```python
from build123d import *

# Parameters (mm, degrees)
SALIENTE_EXTRUIR1_DEPTH = 10
REDONDEO1_R             = 10
REDONDEO2_R             = 10
CROQUIS2_R              = 2
CORTAR_EXTRUIR1_DEPTH   = 10


with BuildPart() as part:
    # Croquis1 → Saliente-Extruir1 (new body)
    with BuildSketch(Plane.XY):
        with BuildLine():
            Line((-15.183023411, 0), (15.183023411, 0))
            ThreePointArc((15.183023411, 0), (22.254091223, -2.928932188), (25.183023411, -10))
            Line((25.183023411, -10), (25.183023411, -16))
            ThreePointArc((25.183023411, -16), (22.254091223, -23.071067812), (15.183023411, -26))
            Line((15.183023411, -26), (12.183023411, -26))
            Line((12.183023411, -26), (12.183023411, -33))
            Line((12.183023411, -33), (25.183023411, -33))
            Line((25.183023411, -33), (32.183023411, -33))
            Line((32.183023411, -33), (32.183023411, 7))
            Line((32.183023411, 7), (32.183023411, 29.676278345))
            Line((32.183023411, 29.676278345), (19.078273373, 35.787123646))
            Line((19.078273373, 35.787123646), (16.119945541, 29.442969137))
            Line((16.119945541, 29.442969137), (25.183023411, 25.216786519))
            Line((25.183023411, 25.216786519), (23.183023411, 20.927772678))
            Line((23.183023411, 20.927772678), (25.183023411, 20.927772678))
            Line((25.183023411, 20.927772678), (25.183023411, 12))
            ThreePointArc((25.183023411, 12), (23.718557317, 8.464466094), (20.183023411, 7))
            Line((20.183023411, 7), (18.68839635, 7))
            Line((18.68839635, 7), (18.68839635, 11.289013841))
            Line((18.68839635, 11.289013841), (16.68839635, 7))
            Line((16.68839635, 7), (12.399382509, 9))
            Line((12.399382509, 9), (12.399382509, 7))
            Line((12.399382509, 7), (-15.183023411, 7))
            ThreePointArc((-15.183023411, 7), (-22.254091223, 9.928932188), (-25.183023411, 17))
            Line((-25.183023411, 17), (-25.183023411, 20.524963692))
            ThreePointArc((-25.183023411, 20.524963692), (-24.011450536, 23.353390817), (-21.183023411, 24.524963692))
            Line((-21.183023411, 24.524963692), (-20.89400957, 24.524963692))
            Line((-20.89400957, 24.524963692), (-25.183023411, 26.524963692))
            Line((-25.183023411, 26.524963692), (-16.68839635, 44.741750212))
            Line((-16.68839635, 44.741750212), (-7.62531848, 40.515567594))
            Line((-7.62531848, 40.515567594), (-4.666990648, 46.859722104))
            Line((-4.666990648, 46.859722104), (-20.074223027, 54.044232553))
            Line((-20.074223027, 54.044232553), (-32.183023411, 28.076826331))
            Line((-32.183023411, 28.076826331), (-32.183023411, 7))
            Line((-32.183023411, 7), (-32.183023411, -33))
            Line((-32.183023411, -33), (-25.183023411, -33))
            Line((-25.183023411, -33), (-12.183023411, -33))
            Line((-12.183023411, -33), (-12.183023411, -26))
            Line((-12.183023411, -26), (-15.183023411, -26))
            ThreePointArc((-15.183023411, -26), (-22.254091223, -23.071067812), (-25.183023411, -16))
            Line((-25.183023411, -16), (-25.183023411, -10))
            ThreePointArc((-25.183023411, -10), (-22.254091223, -2.928932188), (-15.183023411, 0))
        make_face()
    extrude(amount=SALIENTE_EXTRUIR1_DEPTH)

    # Redondeo1
    # the kernel refuses this fillet: 10 mm, written as the material it adds along each edge
    with BuildSketch(Plane(origin=(18.68839635, 7, 0), x_dir=(0, 1, 0), z_dir=(0, 0, 1))) as redondeo1_piece_1_section:
        with BuildLine():
            CenterArc((10, -8.208814597), REDONDEO1_R, 124.826871163, 55.173128837)
            Line((0, -8.208814597), (-0.2, -8.208814597))
            Line((-0.2, -8.208814597), (-0.2, 0))
            Line((-0.2, 0), (0, 0.2))
            ThreePointArc((0, 0.2), (2.144506921, 0.2), (4.174794118, 0.164176292))
            Line((4.174794118, 0.164176292), (4.289013841, 0))
        make_face()
    redondeo1_piece_1 = extrude(amount=10, mode=Mode.PRIVATE)
    redondeo1_piece_1 = split(redondeo1_piece_1, bisect_by=Plane(origin=(17.840933122, 9.471623083, 5), z_dir=(0.9063077870366527, -0.4226182617406938, 0)), keep=Keep.TOP, mode=Mode.PRIVATE)
    add(redondeo1_piece_1)
    with BuildSketch(Plane(origin=(12.399382509, 7, 0), x_dir=(-1, 0, 0), z_dir=(0, 0, 1))) as redondeo1_piece_2:
        with BuildLine():
            CenterArc((6, -10), REDONDEO1_R, 90, 36.869897646)
            Line((0, -2), (-0.12, -1.84))
            ThreePointArc((-0.12, -1.84), (-0.2, -1), (-0.2, 0))
            Line((-0.2, 0), (0, 0.2))
            Line((0, 0.2), (6, 0.2))
            Line((6, 0.2), (6, 0))
        make_face()
    extrude(amount=10)

    # Redondeo2
    # the kernel refuses this fillet: 10 mm, written as the material it adds along each edge
    with BuildSketch(Plane(origin=(25.183023411, 20.927772678, 0), x_dir=(-1, 0, 0), z_dir=(0, 0, 1))) as redondeo2_piece_1:
        with BuildLine():
            CenterArc((10, 6), REDONDEO2_R, 180, 36.869897646)
            Line((0, 6), (-0.2, 6))
            Line((-0.2, 6), (-0.2, 0))
            Line((-0.2, 0), (0, -0.2))
            ThreePointArc((0, -0.2), (1, -0.2), (1.84, -0.12))
            Line((1.84, -0.12), (2, 0))
        make_face()
    extrude(amount=10)

    # Croquis2 → Cortar-Extruir1 (cut)
    with BuildSketch(Plane.XZ.offset(33)):
        with Locations(Location((-17.183023411, 5, 0), (0, 0, 270))):
            Circle(CROQUIS2_R)
        with Locations(Location((17.183023411, 5, 0), (0, 0, 270))):
            Circle(CROQUIS2_R)
    extrude(amount=-CORTAR_EXTRUIR1_DEPTH, mode=Mode.SUBTRACT)


solid = part.part
```
Geometry: final body of the model. Coordinates: model frame, mm. A direction names the side the tool comes from. Coordinates: 2 decimals unless noted, no trailing zeros. Order: outer loops, then holes, each group sorted by start corner. A loop starts at its lowest first (then second) coordinate and runs counter-clockwise, first axis right, second up. Notation, with made-up numbers: M 21,75 L 54,75 A25 cw 54,95 Z; hole C -5,7 d5. An arc over 180 degrees is marked long. Answer in a Markdown table with one row per item. Add a question column.
Q1. Mould query, pull axis X, two halves, no side actions, for faces 1 (the flat face through (22, -33, 5)), 2 (the flat face through (-21, 35.5, 4.9)), 3 (the flat face through (-6, 44, 5)). Classes: released by +X, released by -X, zero draft, split by the parting line, or undercut.
Q2. Section query D-D on y = 48.5. Return the cut outline in (x, z).
Q3. Line query: L1, parallel to X at y = -28.25, z = 5; L2, parallel to X at y = -11.5, z = 2.75; L3, parallel to Y at x = -24, z = 5.25. Output: solid intervals per line, ascending.
Q4. Section query A-A on y = -8. Return the cut outline in (x, z), and give its area (3 significant figures).
Q5. Reachability of faces 4 (the flat face through (-32.183, -2, 5)), 5 (the flat face through (25.183, -13, 5)), 6 (the cylindrical face through (9.52, 7.5, 4.93)), 7 (the cylindrical face through (-19.135, -29.136, 5.434)) from +Z, -Z, +X, -X, +Y, -Y: full face, straight path, thin tool, end or side. Return the list, or none.
Q6. Section query B-B on y = -23. Return the cut outline in (x, z).
Q7. Contact query for flat-ended pins moving along their axis: P1, Ø3.5, axis at x = -13.5, z = 7.5, coming from the +Y side; P2, Ø3, axis at x = 17.18, z = 5, coming from the -Y side; P3, Ø0.9, axis at x = 13.5, z = 3.5, coming from the +Y side; P4, Ø5, axis at x = -19, z = 8, coming from the +Y side. Output: stop coordinate, or through.
Q8. Section query C-C on x = 1. Return the cut outline in (y, z), and give its area (3 significant figures).
Completed:
| question | item | result |
|---|---|---|
| 1 | face 1 | zero draft |
| 1 | face 2 | undercut |
| 1 | face 3 | released by +X |
| 2 | outline | M -22.66,0 L -8.18,0 L -8.18,10 L -22.66,10 Z |
| 3 | L1 | x = -32.18 to -19.18, -15.18 to -12.18, 12.18 to 15.18, 19.18 to 32.18 |
| 3 | L2 | x = -32.18 to -25.18, 25.18 to 32.18 |
| 3 | L3 | y = -33 to -20.72, -5.28 to 12.28, 23.36 to 25.97, 29.06 to 45.63 |
| 4 | outline | M -32.18,0 L -24.98,0 L -24.98,10 L -32.18,10 Z; M 24.98,0 L 32.18,0 L 32.18,10 L 24.98,10 Z |
| 4 | area | 144 mm2 |
| 5 | face 4 | +Z, -Z, -X, +Y, -Y |
| 5 | face 5 | +Z, -Z |
| 5 | face 6 | +Z, -Z, +Y |
| 5 | face 7 | -Y |
| 6 | outline | M -32.18,0 L -22.32,0 L -22.32,10 L -32.18,10 Z; M 22.32,0 L 32.18,0 L 32.18,10 L 22.32,10 Z |
| 7 | P1 | stops at y = 51.79 |
| 7 | P2 | stops at y = -0.63 |
| 7 | P3 | stops at y = 8.7 |
| 7 | P4 | stops at y = 54.04 |
| 8 | outline | M 0,0 L 7,0 L 7,10 L 0,10 Z |
| 8 | area | 70.0 mm2 |
